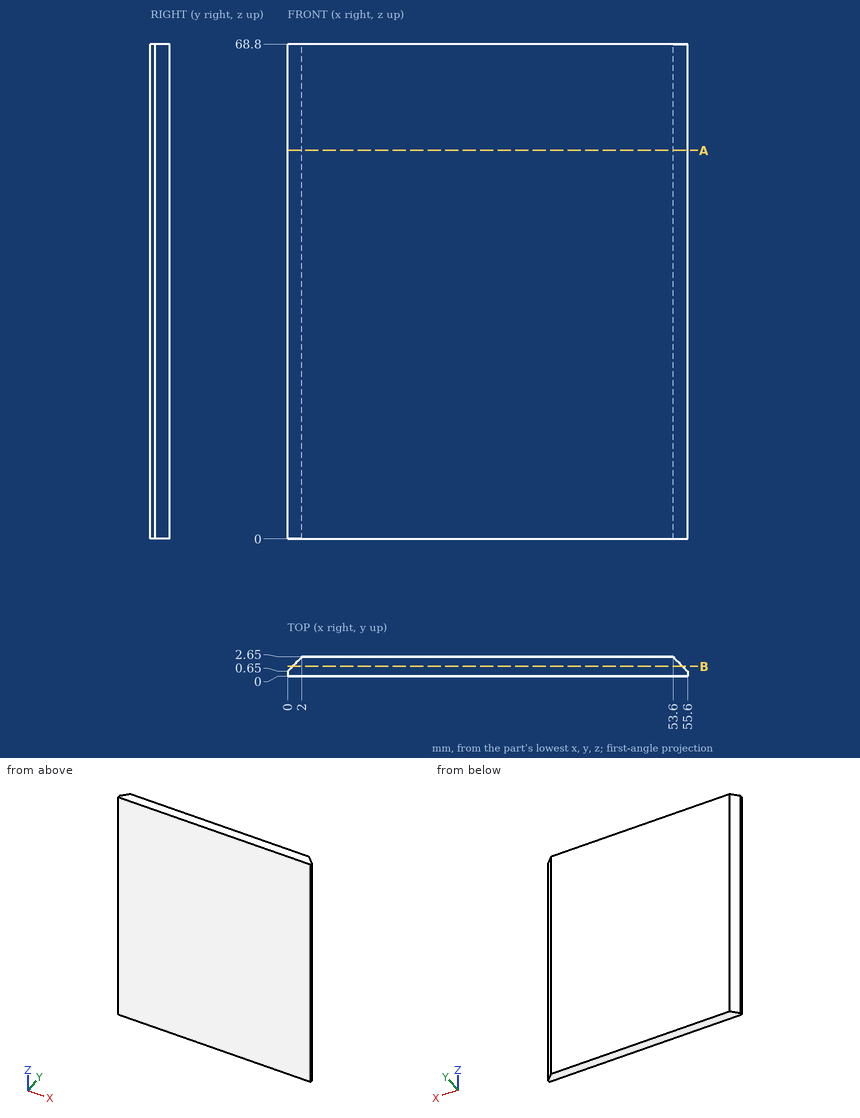
Geometry check sheet. Reference: drawing and pictorial views, mm from the part's lowest x, y, z. Coordinates: 2 decimals unless noted, no trailing zeros. Write each loop counter-clockwise with the first axis right and the second up, starting at its lowest first coordinate (ties: lowest second). Pieces come first, ordered by that corner, then holes. Notation, with made-up numbers: M -11.5,74.5 L -5.5,74.5 A19 ccw -5.5,93.5 Z; hole C -37.75,-14.75 d1. An arc over 180 degrees is marked long. Write item = value, one per line. Start each with the question number.
1. Thickness scan on probe 1 along X at (y, z) = (1.05, 57.5); probe 2 along X at (y, z) = (0.85, 30). Record the ranges inside material, lowest first.
2. Sectioned sample at B-B (y = 1.35). Record the cut outline in (x, z), then the cut area to 3 significant figures.
3. Sectioned sample at A-A (z = 54). Record the cut outline in (x, y).
The answers:
q1.probe_1 = 0.4 to 55.2
q1.probe_2 = 0.2 to 55.4
q2.outline = M 0.7,0 L 54.9,0 L 54.9,68.8 L 0.7,68.8 Z
q2.area = 3,730 mm²
q3.outline = M 0,0 L 55.6,0 L 55.6,0.65 L 53.6,2.65 L 2,2.65 L 0,0.65 Z
